from build123d import *

# Parameters (mm, degrees)
BOSS_EXTRUDE1_DEPTH     = 3.175
SKETCH2_R               = 38.1
CUT_EXTRUDE1_DEPTH      = 1
CUT_EXTRUDE1_DEPTH_BACK = 4.175
SKETCH3_R               = 3.81
CUT_EXTRUDE2_DEPTH      = 4.175
SKETCH4_W               = 12.7
SKETCH4_H               = 19.05
SKETCH4_H_2             = 25.4
CUT_EXTRUDE3_DEPTH      = 4.175


with BuildPart() as part:
    # Sketch1 → Boss-Extrude1 (new body)
    with BuildSketch(Plane(origin=(0, 0, 0), x_dir=(1, 0, 0), z_dir=(0, 1, 0))):
        Polygon((63.126146906, 152.4), (-63.126146906, 152.4), (-152.4, 63.126146906), (-152.4, -63.126146906), (-63.126146906, -152.4), (63.126146906, -152.4), (152.4, -63.126146906), (152.4, 63.126146906), align=None)
    extrude(amount=BOSS_EXTRUDE1_DEPTH)

    # Sketch2 → Cut-Extrude1 (cut, two sides)
    with BuildSketch(Plane(origin=(0, 3.175, 0), x_dir=(1, 0, 0), z_dir=(0, 1, 0))) as cut_extrude1_sk:
        Circle(SKETCH2_R)
    extrude(amount=CUT_EXTRUDE1_DEPTH, mode=Mode.SUBTRACT)
    extrude(cut_extrude1_sk.sketch, amount=-CUT_EXTRUDE1_DEPTH_BACK, mode=Mode.SUBTRACT)

    # Sketch3 → Cut-Extrude2 (cut, through all)
    with BuildSketch(Plane(origin=(0, 3.175, 0), x_dir=(1, 0, 0), z_dir=(0, 1, 0))):
        with Locations((44.463441276, -107.344242958)):
            Circle(SKETCH3_R)
        with Locations((-44.463441276, -107.344242958)):
            Circle(SKETCH3_R)
        with Locations((-107.344242958, -44.463441276)):
            Circle(SKETCH3_R)
        with Locations((-107.344242958, 44.463441276)):
            Circle(SKETCH3_R)
        with Locations((-44.463441276, 107.344242958)):
            Circle(SKETCH3_R)
        with Locations((44.463441276, 107.344242958)):
            Circle(SKETCH3_R)
        with Locations((107.344242958, 44.463441276)):
            Circle(SKETCH3_R)
        with Locations((107.344242958, -44.463441276)):
            Circle(SKETCH3_R)
    extrude(amount=-CUT_EXTRUDE2_DEPTH, mode=Mode.SUBTRACT)

    # Sketch4 → Cut-Extrude3 (cut, through all)
    with BuildSketch(Plane(origin=(0, 3.175, 0), x_dir=(1, 0, 0), z_dir=(0, 1, 0))):
        with Locations((-38.1, 0)):
            Rectangle(SKETCH4_W, SKETCH4_H)
        with Locations((38.1, 0)):
            Rectangle(SKETCH4_W, SKETCH4_H)
        with Locations((0, 38.1)):
            Rectangle(SKETCH4_W, SKETCH4_H_2)
    extrude(amount=-CUT_EXTRUDE3_DEPTH, mode=Mode.SUBTRACT)


solid = part.part
The listing builds one solid part. Answer for the finished solid, in the listing's coordinates (mm). A direction names the side the tool comes from. Give positions to 0.01 mm unless a question says otherwise; leave off trailing zeros. Order: outer loops, then holes, each group sorted by start corner. A loop starts at its lowest first (then second) coordinate and runs counter-clockwise, first axis right, second up. Notation, with made-up numbers: (87, 85) - (125, 85) arc R21 ccw to (125, 95) - close; hole circle Ø11 at (55, 68). An arc over 180 degrees is marked (long way). Answer as CSV lines item,"result".
Q1. A cutting plane is placed at A-A, the plane x = 21. Determine the outline of the cut face in (y, z) (3 decimals).
Answer key:
outline,"(0, -152.4) - (3.175, -152.4) - (3.175, -31.79) - (0, -31.79) - close; (0, 31.79) - (3.175, 31.79) - (3.175, 152.4) - (0, 152.4) - close"
Q2. Which of the six approach directions +Z, -Z, +X, -X, +Y, -Y give full straight-line access (tool end or side, diameter ignored) to faces 4 (the face through (25.99, 1.61, -27.86)), 5 (the face through (108.388, 1.565, -107.138))?
Answer key:
face 4,"+Y, -Y"
face 5,"-Z, +X, +Y, -Y"
Q3. A cutting plane is placed at D-D, the plane z = 125.5. Determine the outline of the cut face in (x, y) (3 decimals), and give its area (3 significant figures).
Answer key:
outline,"(-90.026, 0) - (90.026, 0) - (90.026, 3.175) - (-90.026, 3.175) - close"
area,"572 mm^2"
Q4. Each of these flat-tipped pins is pushed along its axis until it touches: pin 1 Ø1.5 at (y, z) = (1, 77.5) entering from -X; pin 2 Ø7 at (x, z) = (-107.34, 44.46) entering from +Y; pin 3 Ø1 at (y, z) = (2, -85.5) entering from -X. Where does it stop, or does it pass through?
Answer key:
pin 1,"stops at x = -138.78"
pin 2,"passes through"
pin 3,"stops at x = -130.53"
Q5. Determine the mould class of faces 1 (the face through (-107.138, 1.565, -108.388)), 2 (the face through (107.138, 1.565, 108.388)), 3 (the face through (41.655, 1.61, 104.769)) for opening direction Z: pulls with the +Z half, pulls with the -Z half, needs draft (parallel to the pull), parting line crosses it, or undercut.
Answer key:
face 1,"pulls with the -Z half"
face 2,"pulls with the +Z half"
face 3,"undercut"
Q6. A cutting plane is placed at B-B, the plane y = 2.6. Count the separate pieces of the cut face and the enclosed holes in it, and give its area (3 significant figures).
Answer key:
separate pieces,"1"
enclosed holes,"9"
area,"71,600 mm^2"
Q7. A cutting plane is placed at C-C, the plane z = -97. Determine the outline of the cut face in (x, y) (3 decimals), and give its area (3 significant figures).
Answer key:
outline,"(-118.526, 0) - (118.526, 0) - (118.526, 3.175) - (-118.526, 3.175) - close"
area,"753 mm^2"
Q8. Straight lines are drawn through the part: L1, parallel to Z at x = 44.5, y = 0.2; L2, parallel to Z at x = 37.5, y = 0.5 (3 decimals); L3, parallel to X at y = 2.15, z = 109. For each, find the intervals that lie inside material, in ascending order.
Answer key:
L1,"z = -152.4 to -111.15, -103.53 to 103.53, 111.15 to 152.4"
L2,"z = -152.4 to -9.525, 9.525 to 152.4"
L3,"x = -106.53 to -47.89, -41.03 to 41.03, 47.89 to 106.53"
